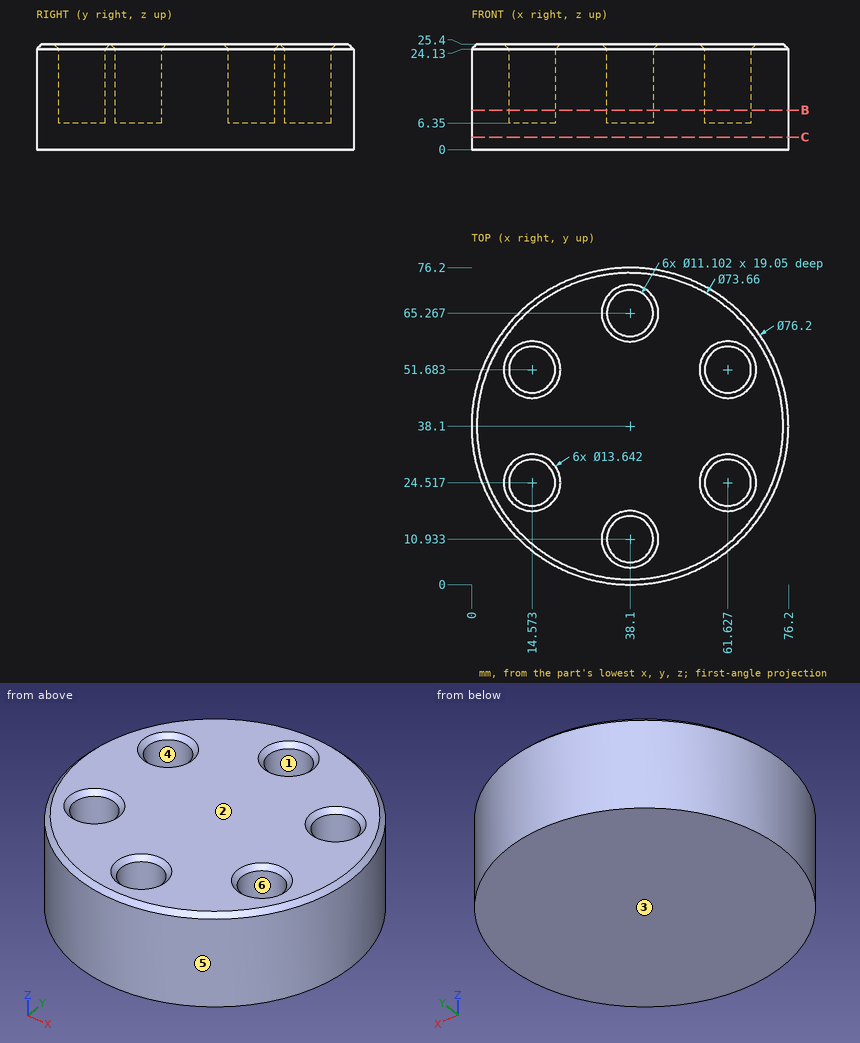
Here's the drawing with two shaded views (mm, measured from the low corner). I have some questions. A direction names the side the tool comes from. Round coordinates to 2 decimals unless told otherwise and drop trailing zeros. Order: outer loops, then holes, each group sorted by start corner. A loop starts at its lowest first (then second) coordinate and runs counter-clockwise, first axis right, second up. Notation, with made-up numbers: (28.5, 25) -> (63.5, 25) arc R18 cw to (63.5, 41) -> close; hole circle Ø7 at (8.5, 60.5). An arc over 180 degrees is marked (long way). Use a Markdown table: item, result. Add a question column.
(1) Suppose I cut it at B-B, the plane z = 9.5. Please give me the cut outline in (x, y).
(2) For the marked faces 1 and 2, which set-ups out of +Z, -Z, +X, -X, +Y, -Y let a thin tool reach every point of the face, with its end or its side?
(3) If we mould it in two halves opening along Y, with no side actions, what happens to the marked faces 3, 4, 5 and 6? For each: released by +Y, released by -Y, zero draft, split by the parting line, or undercut.
(4) For pin 1 Ø9 at (x, y) = (59.5, 26.5) entering from +Z; pin 2 Ø9 at (x, y) = (38, 11.5) entering from +Z; pin 3 Ø10 at (y, z) = (13.5, 7.5) entering from +X; pin 4 Ø5 at (y, z) = (30.5, 9.5) entering from +X, each with a flat end and sliding along its axis, tell me the tip position at first contact or that it passes through.
(5) Suppose I cut it at C-C, the plane z = 3. Please give me the cut outline in (x, y), and give its area (3 significant figures).
(6) I need wall thicknesses on line 1 along Y through (x, z) = (38.1, 17.75) (1 decimal); line 2 along X through (y, z) = (47.5, 16.5) (1 decimal); line 3 along Y through (x, z) = (63.5, 10.25). Which ranges of each line are inside material? Lowest first, please.
Verdict:
| question | item | result |
|---|---|---|
| 1 | outline | circle Ø76.2 at (38.1, 38.1); hole circle Ø11.1 at (14.57, 24.52); hole circle Ø11.1 at (14.57, 51.68); hole circle Ø11.1 at (38.1, 10.93); hole circle Ø11.1 at (38.1, 65.27); hole circle Ø11.1 at (61.63, 24.52); hole circle Ø11.1 at (61.63, 51.68) |
| 2 | face 1 | +Z |
| 2 | face 2 | +Z, +X, -X, +Y, -Y |
| 3 | face 3 | zero draft |
| 3 | face 4 | undercut |
| 3 | face 5 | split by the parting line |
| 3 | face 6 | undercut |
| 4 | pin 1 | z = 25.4 |
| 4 | pin 2 | z = 6.35 |
| 4 | pin 3 | x = 70.77 |
| 4 | pin 4 | x = 75.86 |
| 5 | outline | circle Ø76.2 at (38.1, 38.1) |
| 5 | area | 4,560 mm2 |
| 6 | line 1 | 0 to 5.4, 16.5 to 59.7, 70.8 to 76.2 |
| 6 | line 2 | 1.2 to 10.9, 18.2 to 58, 65.3 to 75 |
| 6 | line 3 | 9.7 to 19.29, 29.74 to 46.46, 56.91 to 66.5 |
